from build123d import *

# Parameters (mm, degrees)
BOSS_EXTRUDE1_OUTLINE_R   = 1
BOSS_EXTRUDE1_OUTLINE_W   = 5
BOSS_EXTRUDE1_OUTLINE_H   = 5
BOSS_EXTRUDE1_OUTLINE_R_2 = 1.5
BOSS_EXTRUDE1_OUTLINE_R_3 = 4.05
BOSS_EXTRUDE1_DEPTH       = 2
CONG_1_R                  = 5


# Read off the part's stored shape, not the designer's step: Boss-Extrude1
with BuildPart() as part:
    # Boss-Extrude1 outline → Boss-Extrude1 (new body)
    with BuildSketch(Plane.XY):
        with BuildLine():
            Line((51, -11.7), (51, 11.7))
            Line((51, 11.7), (0, 11.7))
            ThreePointArc((0, 11.7), (-11.7, 0), (0, -11.7))
            Line((0, -11.7), (51, -11.7))
        make_face()
        with Locations((0, -7)):
            Circle(BOSS_EXTRUDE1_OUTLINE_R, mode=Mode.SUBTRACT)
        with Locations((-3.5, -6.062177826)):
            Circle(BOSS_EXTRUDE1_OUTLINE_R, mode=Mode.SUBTRACT)
        with Locations((3.5, -6.062177826)):
            Circle(BOSS_EXTRUDE1_OUTLINE_R, mode=Mode.SUBTRACT)
        with Locations((-6.062177826, -3.5)):
            Circle(BOSS_EXTRUDE1_OUTLINE_R, mode=Mode.SUBTRACT)
        with Locations((6.062177826, -3.5)):
            Circle(BOSS_EXTRUDE1_OUTLINE_R, mode=Mode.SUBTRACT)
        with Locations((30.5, -5)):
            Rectangle(BOSS_EXTRUDE1_OUTLINE_W, BOSS_EXTRUDE1_OUTLINE_H, mode=Mode.SUBTRACT)
        with Locations((38, -5)):
            Circle(BOSS_EXTRUDE1_OUTLINE_R_2, mode=Mode.SUBTRACT)
        with Locations((45.5, -5)):
            Rectangle(BOSS_EXTRUDE1_OUTLINE_W, BOSS_EXTRUDE1_OUTLINE_H, mode=Mode.SUBTRACT)
        with Locations((-7, 0)):
            Circle(BOSS_EXTRUDE1_OUTLINE_R, mode=Mode.SUBTRACT)
        Circle(BOSS_EXTRUDE1_OUTLINE_R_3, mode=Mode.SUBTRACT)
        with Locations((-6.062177826, 3.5)):
            Circle(BOSS_EXTRUDE1_OUTLINE_R, mode=Mode.SUBTRACT)
        with Locations((7, 0)):
            Circle(BOSS_EXTRUDE1_OUTLINE_R, mode=Mode.SUBTRACT)
        with Locations((6.062177826, 3.5)):
            Circle(BOSS_EXTRUDE1_OUTLINE_R, mode=Mode.SUBTRACT)
        with Locations((-3.5, 6.062177826)):
            Circle(BOSS_EXTRUDE1_OUTLINE_R, mode=Mode.SUBTRACT)
        with Locations((0, 7)):
            Circle(BOSS_EXTRUDE1_OUTLINE_R, mode=Mode.SUBTRACT)
        with Locations((3.5, 6.062177826)):
            Circle(BOSS_EXTRUDE1_OUTLINE_R, mode=Mode.SUBTRACT)
        with Locations((30.5, 5)):
            Rectangle(BOSS_EXTRUDE1_OUTLINE_W, BOSS_EXTRUDE1_OUTLINE_H, mode=Mode.SUBTRACT)
        with Locations((38, 5)):
            Circle(BOSS_EXTRUDE1_OUTLINE_R_2, mode=Mode.SUBTRACT)
        with Locations((45.5, 5)):
            Rectangle(BOSS_EXTRUDE1_OUTLINE_W, BOSS_EXTRUDE1_OUTLINE_H, mode=Mode.SUBTRACT)
    extrude(amount=BOSS_EXTRUDE1_DEPTH)

    # Congé1
    cong_1_edges = [part.edges().sort_by_distance(p)[0] for p in [
        (51, 11.7, 1),
        (51, -11.7, 1),
    ]]
    fillet(cong_1_edges, radius=CONG_1_R)


solid = part.part
Could you check a few things on this model? Use its own coordinates, in mm. A direction names the side the tool comes from. Give positions to 0.01 mm unless a question says otherwise; leave off trailing zeros. Loops run counter-clockwise (first coordinate to the right, second up) from the corner with the lowest first, then second, coordinate; pieces in that order, holes last. Notation, with made-up numbers: (-5, -17) -> (37, -17) arc R17 cw to (37, 6) -> close; hole circle Ø10 at (81, 14.25). An arc over 180 degrees is marked (long way). Return JSON: item names as keys, results as strings.
Item 1: I'm going to push flat-ended pins straight in: pin 1 (1 mm diameter, centred on y = -8.5, z = 1, fed in from +X); pin 2 (1 mm diameter, centred on y = 4.5, z = 1, fed in from -X) (3 decimals). Where does each tip first touch, or does it pass through?
Geometry results:
{"pin 1": "stops at x = 50.83", "pin 2": "stops at x = -10.995"}
Item 2: Which directions (+Z, -Z, +X, -X, +Y, -Y) give clear straight access to the entire face, cutting with the end or side of a thin tool? Please do faces 1 (the flat face through (45, -2.5, 1)), 2 (the cylindrical face through (-11.697, 0.257, 0.986)).
Geometry results:
{"face 1": "+Z, -Z", "face 2": "+Z, -Z, -X"}
Item 3: If we section it at A-A on x = 38: List the corners of the cut face in (y, z) for me.
Geometry results:
{"outline": "(-11.7, 0) -> (-6.5, 0) -> (-6.5, 2) -> (-11.7, 2) -> close; (-3.5, 0) -> (3.5, 0) -> (3.5, 2) -> (-3.5, 2) -> close; (6.5, 0) -> (11.7, 0) -> (11.7, 2) -> (6.5, 2) -> close"}
Item 4: We'd pull the mould along X, two halves only. Please class faces 3 (the cylindrical face through (49.57, -10.2, 1.01)), 4 (the flat face through (23, 11.7, 1)), 5 (the flat face through (30, 7.5, 1)): +X half, -X half, draft (parallel to the pull), parting line (faces both ways), or undercut.
Geometry results:
{"face 3": "+X half", "face 4": "draft", "face 5": "undercut"}
Item 5: If we section it at C-C on z = 1.6: Count the separate pieces of the cut face and the enclosed holes in it, plus the area to 3 significant figures.
Geometry results:
{"separate pieces": "1", "enclosed holes": "19", "area": "1,190 mm²"}
Item 6: I need wall thicknesses on L1, parallel to Y at x = 38, z = 0.65; L2, parallel to Y at x = 37, z = 0.25; L3, parallel to X at y = 2.75, z = 0.85. Which ranges of each line are inside material? Lowest first, please. Write a range as from..to.
Geometry results:
{"L1": "y = -11.7..-6.5, -3.5..3.5, 6.5..11.7", "L2": "y = -11.7..-6.12, -3.88..3.88, 6.12..11.7", "L3": "x = -11.37..-6.72, -5.4..-2.97, 2.97..5.4, 6.72..28, 33..43, 48..51"}
Item 7: If we section it at B-B on x = -3.5: List the corners of the cut face in (y, z) for me.
Geometry results:
{"outline": "(-11.16, 0) -> (-7.06, 0) -> (-7.06, 2) -> (-11.16, 2) -> close; (-5.06, 0) -> (-2.04, 0) -> (-2.04, 2) -> (-5.06, 2) -> close; (2.04, 0) -> (5.06, 0) -> (5.06, 2) -> (2.04, 2) -> close; (7.06, 0) -> (11.16, 0) -> (11.16, 2) -> (7.06, 2) -> close"}
